from build123d import *

# Parameters (mm, degrees)
BOSS_EXTRUDE1_DEPTH = 6
SKETCH3_R           = 2.2
SKETCH3_R_2         = 1.7
CUT_EXTRUDE1_DEPTH  = 263.645900158
SKETCH9_R           = 1.5
CUT_EXTRUDE7_DEPTH  = 263.645900158
SKETCH10_R          = 2
CUT_EXTRUDE8_DEPTH  = 263.645900158
SKETCH11_R          = 1.5621
CUT_EXTRUDE9_DEPTH  = 263.645900158


with BuildPart() as part:
    # Sketch2 → Boss-Extrude1 (new body)
    with BuildSketch(Plane.XY):
        with BuildLine():
            ThreePointArc((14.643567385, -34.35021296), (17.582213792, -26.298472933), (14.643567385, -18.246732906))
            ThreePointArc((14.643567385, -18.246732906), (1.271257198, 11.050387409), (4.97338396, 43.041545498))
            ThreePointArc((4.97338396, 43.041545498), (-4.554295145, 63.052831737), (-23.608507858, 51.731823656))
            ThreePointArc((-23.608507858, 51.731823656), (-56.417786208, 24.999486038), (-89.227064559, 51.731823656))
            ThreePointArc((-89.227064559, 51.731823656), (-103.917786208, 63.701527067), (-118.608507858, 51.731823656))
            ThreePointArc((-118.608507858, 51.731823656), (-151.417786208, 24.999486038), (-184.227064559, 51.731823656))
            ThreePointArc((-184.227064559, 51.731823656), (-203.236955544, 63.06623299), (-212.843634986, 43.127414061))
            ThreePointArc((-212.843634986, 43.127414061), (-211.27621055, 10.502270588), (-230.186855149, -16.129370872))
            ThreePointArc((-230.186855149, -16.129370872), (-235.417786208, -26.298472933), (-230.186855149, -36.467574994))
            ThreePointArc((-230.186855149, -36.467574994), (-211.27621055, -63.099216454), (-212.843634986, -95.724359927))
            ThreePointArc((-212.843634986, -95.724359927), (-203.236955544, -115.663178856), (-184.227064559, -104.328769522))
            ThreePointArc((-184.227064559, -104.328769522), (-151.417786208, -77.596431904), (-118.608507858, -104.328769522))
            ThreePointArc((-118.608507858, -104.328769522), (-103.917786208, -116.298472933), (-89.227064559, -104.328769522))
            ThreePointArc((-89.227064559, -104.328769522), (-56.417786208, -77.596431904), (-23.608507858, -104.328769522))
            ThreePointArc((-23.608507858, -104.328769522), (-4.554295145, -115.649777603), (4.97338396, -95.638491364))
            ThreePointArc((4.97338396, -95.638491364), (1.271257198, -63.647333275), (14.643567385, -34.35021296))
        make_face()
    extrude(amount=BOSS_EXTRUDE1_DEPTH)

    # Sketch3 → Cut-Extrude1 (cut, through all)
    with BuildSketch(Plane.XY.offset(6)):
        with Locations((-222.917786208, -26.298472933)):
            Circle(SKETCH3_R)
        with Locations((-198.917786208, -101.298472933)):
            Circle(SKETCH3_R)
        with Locations((-103.917786208, -101.298472933)):
            Circle(SKETCH3_R)
        with Locations((-8.917786208, -101.298472933)):
            Circle(SKETCH3_R)
        with Locations((-5.417786208, -10.298472933)):
            Circle(SKETCH3_R_2)
        with Locations((-5.417786208, -42.298472933)):
            Circle(SKETCH3_R_2)
        with Locations((2.582213792, -42.298472933)):
            Circle(SKETCH3_R_2)
        with Locations((2.582213792, -10.298472933)):
            Circle(SKETCH3_R_2)
        with Locations((-8.917786208, 48.701527067)):
            Circle(SKETCH3_R)
        with Locations((-103.917786208, 48.701527067)):
            Circle(SKETCH3_R)
        with Locations((-198.917786208, 48.701527067)):
            Circle(SKETCH3_R)
    extrude(amount=-CUT_EXTRUDE1_DEPTH, mode=Mode.SUBTRACT)

    # Sketch9 → Cut-Extrude7 (cut, through all)
    with BuildSketch(Plane.XY.offset(6)):
        with Locations((-103.99500987, 12.281928067)):
            Circle(SKETCH9_R)
        with Locations((-103.99500987, 2.917326067)):
            Circle(SKETCH9_R)
    extrude(amount=-CUT_EXTRUDE7_DEPTH, mode=Mode.SUBTRACT)

    # Sketch10 → Cut-Extrude8 (cut, through all)
    with BuildSketch(Plane.XY.offset(6)):
        with Locations((-4.70262179, 15.909627067)):
            Circle(SKETCH10_R)
        with Locations((-4.70262179, -0.590372933)):
            Circle(SKETCH10_R)
        with Locations((-73.95262179, 15.909627067)):
            Circle(SKETCH10_R)
        with Locations((-73.95262179, -0.590372933)):
            Circle(SKETCH10_R)
    extrude(amount=-CUT_EXTRUDE8_DEPTH, mode=Mode.SUBTRACT)

    # Sketch11 → Cut-Extrude9 (cut, through all)
    with BuildSketch(Plane.XY.offset(6)):
        with Locations((-23.040186208, -9.130372933)):
            Circle(SKETCH11_R)
        with Locations((-23.040186208, -57.466572933)):
            Circle(SKETCH11_R)
        with Locations((-105.666386208, -9.130372933)):
            Circle(SKETCH11_R)
        with Locations((-98.173386208, -57.466572933)):
            Circle(SKETCH11_R)
    extrude(amount=-CUT_EXTRUDE9_DEPTH, mode=Mode.SUBTRACT)


solid = part.part
Geometry check sheet. Reference: the model listing, model coordinates, mm. Coordinates: 2 decimals unless noted, no trailing zeros. Order: outer loops, then holes, each group sorted by start corner. A loop starts at its lowest first (then second) coordinate and runs counter-clockwise, first axis right, second up. Notation, with made-up numbers: (39.5, -26) -> (46.5, -26) arc R36 cw to (46.5, 8) -> close; hole circle Ø2 at (64, 85). An arc over 180 degrees is marked (long way). Use a Markdown table: item, result. Add a question column.
1. Mould release check, pull along X, two halves, no side actions. Record for faces 1 (the face through (-111, -25, 6)), 2 (the face through (-104.205, -116.296, 2.958)), 3 (the face through (-235.417, -26.132, 2.958)), 4 (the face through (17.58, -26.42, 2.96)): pulls with the +X half, pulls with the -X half, needs draft (parallel to the pull), parting line crosses it, or undercut.
2. Cross-section at A-A (y = 21.5). Enter the section's corners in (x, z), and give its area (3 significant figures).
3. Material ranges on L1, parallel to X at y = 38, z = 4.3; L2, parallel to X at y = 36, z = 2.9; L3, parallel to X at y = -65.5, z = 2.95, recorded low to high.
4. Cross-section at C-C (z = 1.6). Give the number of separate pieces and of enclosed holes in the cut face, and give its area (3 significant figures).
5. Cross-section at B-B (x = -33.5). Enter the section's corners in (y, z), and give its area (3 significant figures).
6. Go/stop test with flat-tipped pins: pin 1 Ø7 at (x, y) = (-8.92, -101.3) entering from +Z; pin 2 Ø1.5 at (y, z) = (-50, 2.5) entering from +X; pin 3 Ø1 at (y, z) = (41, 3.5) entering from -X; pin 4 Ø1 at (x, z) = (-126.5, 4) entering from -Y. Record where each tip stops, or that it passes through.
Filled sheet:
| question | item | result |
|---|---|---|
| 1 | face 1 | needs draft |
| 1 | face 2 | undercut |
| 1 | face 3 | pulls with the -X half |
| 1 | face 4 | pulls with the +X half |
| 2 | outline | (-209.36, 0) -> (0.55, 0) -> (0.55, 6) -> (-209.36, 6) -> close |
| 2 | area | 1,260 mm2 |
| 3 | L1 | -211.11 to -177.91, -124.92 to -82.91, -29.92 to 3.18 |
| 3 | L2 | -210.59 to -176.24, -126.6 to -81.24, -31.6 to 2.6 |
| 3 | L3 | -210.64 to 1.01 |
| 4 | separate pieces | 1 |
| 4 | enclosed holes | 21 |
| 4 | area | 30,700 mm2 |
| 5 | outline | (-86.66, 0) -> (34.07, 0) -> (34.07, 6) -> (-86.66, 6) -> close |
| 5 | area | 724 mm2 |
| 6 | pin 1 | z = 6 |
| 6 | pin 2 | x = 5.44 |
| 6 | pin 3 | x = -212.22 |
| 6 | pin 4 | y = -89.27 |
